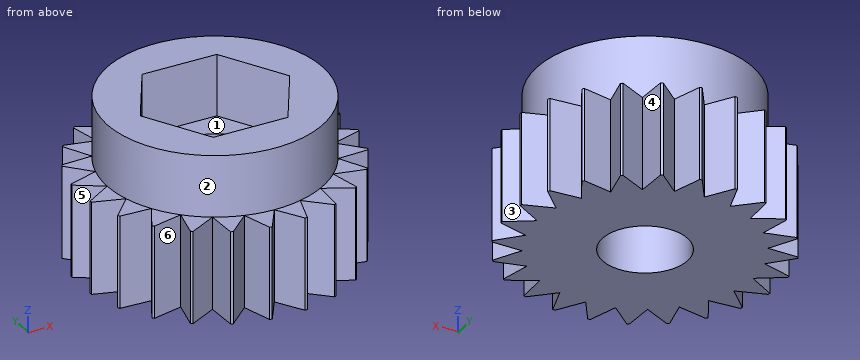
```python
from build123d import *

# Parameters (mm, degrees)
F3_DEPTH = 2.54
F4_R     = 6.6719294198
F5_DEPTH = 25.4


with BuildPart() as f1:
    # F0 (on Front) → F1 (revolve)
    with BuildSketch(Plane.XZ):
        Polygon((-5.56, -6.35), (-1.75, -6.35), (-1.75, 0), (-4.445, 0), (-4.445, -2.54), (-5.56, -2.54), align=None)
    revolve(axis=Axis((0, 0, -3.175), (0, 0, -1)))

    # F2 (on face) → F3 (cut)
    with BuildSketch(Plane.XY):
        Polygon((1.5397931679, 2.667), (-1.5397931679, 2.667), (-3.0795863359, 0), (-1.5397931679, -2.667), (1.5397931679, -2.667), (3.0795863359, 0), align=None)
    extrude(amount=-F3_DEPTH, mode=Mode.SUBTRACT)

    # F4 (on face) → F5 (cut)
    with BuildSketch(Plane.XY.offset(-2.54)):
        Circle(F4_R)
        with BuildLine():
            ThreePointArc((-0.7741932024, 5.5058355302), (-0.7257256287, 5.5124334292), (-0.6772018857, 5.5186046793))
            ThreePointArc((-0.6772018857, 5.5186046793), (0, 5.56), (0.6772018857, 5.5186046793))
            ThreePointArc((0.6772018857, 5.5186046793), (0.7257256287, 5.5124334292), (0.7741932024, 5.5058355302))
            ThreePointArc((0.7741932024, 5.5058355302), (1.4390338908, 5.3705475942), (2.0824467844, 5.1552900394))
            ThreePointArc((2.0824467844, 5.1552900394), (2.1277198839, 5.1367702008), (2.1728283032, 5.1178527885))
            ThreePointArc((2.1728283032, 5.1178527885), (2.78, 4.815101245), (3.3457763761, 4.4406509029))
            ThreePointArc((3.3457763761, 4.4406509029), (3.3847135453, 4.411044572), (3.4233887458, 4.381096837))
            ThreePointArc((3.4233887458, 4.381096837), (3.9315137034, 3.9315137034), (4.381096837, 3.4233887458))
            ThreePointArc((4.381096837, 3.4233887458), (4.411044572, 3.3847135453), (4.4406509029, 3.3457763761))
            ThreePointArc((4.4406509029, 3.3457763761), (4.815101245, 2.78), (5.1178527885, 2.1728283032))
            ThreePointArc((5.1178527885, 2.1728283032), (5.1367702008, 2.1277198839), (5.1552900394, 2.0824467844))
            ThreePointArc((5.1552900394, 2.0824467844), (5.3705475942, 1.4390338908), (5.5058355302, 0.7741932024))
            ThreePointArc((5.5058355302, 0.7741932024), (5.5124334292, 0.7257256287), (5.5186046793, 0.6772018857))
            ThreePointArc((5.5186046793, 0.6772018857), (5.5496415207, 0.339232946), (5.56, 0))
            ThreePointArc((5.56, 0), (5.5496415207, -0.339232946), (5.5186046793, -0.6772018857))
            ThreePointArc((5.5186046793, -0.6772018857), (5.5124334292, -0.7257256287), (5.5058355302, -0.7741932024))
            ThreePointArc((5.5058355302, -0.7741932024), (5.3705475942, -1.4390338908), (5.1552900394, -2.0824467844))
            ThreePointArc((5.1552900394, -2.0824467844), (5.1367702008, -2.1277198839), (5.1178527885, -2.1728283032))
            ThreePointArc((5.1178527885, -2.1728283032), (4.815101245, -2.78), (4.4406509029, -3.3457763761))
            ThreePointArc((4.4406509029, -3.3457763761), (4.411044572, -3.3847135453), (4.381096837, -3.4233887458))
            ThreePointArc((4.381096837, -3.4233887458), (3.9315137034, -3.9315137034), (3.4233887458, -4.381096837))
            ThreePointArc((3.4233887458, -4.381096837), (3.3847135453, -4.411044572), (3.3457763761, -4.4406509029))
            ThreePointArc((3.3457763761, -4.4406509029), (2.78, -4.815101245), (2.1728283032, -5.1178527885))
            ThreePointArc((2.1728283032, -5.1178527885), (2.1277198839, -5.1367702008), (2.0824467844, -5.1552900394))
            ThreePointArc((2.0824467844, -5.1552900394), (1.4390338908, -5.3705475942), (0.7741932024, -5.5058355302))
            ThreePointArc((0.7741932024, -5.5058355302), (0.7257256287, -5.5124334292), (0.6772018857, -5.5186046793))
            ThreePointArc((0.6772018857, -5.5186046793), (0, -5.56), (-0.6772018857, -5.5186046793))
            ThreePointArc((-0.6772018857, -5.5186046793), (-0.7257256287, -5.5124334292), (-0.7741932024, -5.5058355302))
            ThreePointArc((-0.7741932024, -5.5058355302), (-1.4390338908, -5.3705475942), (-2.0824467844, -5.1552900394))
            ThreePointArc((-2.0824467844, -5.1552900394), (-2.1277198839, -5.1367702008), (-2.1728283032, -5.1178527885))
            ThreePointArc((-2.1728283032, -5.1178527885), (-2.78, -4.815101245), (-3.3457763761, -4.4406509029))
            ThreePointArc((-3.3457763761, -4.4406509029), (-3.3847135453, -4.411044572), (-3.4233887458, -4.381096837))
            ThreePointArc((-3.4233887458, -4.381096837), (-3.9315137034, -3.9315137034), (-4.381096837, -3.4233887458))
            ThreePointArc((-4.381096837, -3.4233887458), (-4.411044572, -3.3847135453), (-4.4406509029, -3.3457763761))
            ThreePointArc((-4.4406509029, -3.3457763761), (-4.815101245, -2.78), (-5.1178527885, -2.1728283032))
            ThreePointArc((-5.1178527885, -2.1728283032), (-5.1367702008, -2.1277198839), (-5.1552900394, -2.0824467844))
            ThreePointArc((-5.1552900394, -2.0824467844), (-5.3705475942, -1.4390338908), (-5.5058355302, -0.7741932024))
            ThreePointArc((-5.5058355302, -0.7741932024), (-5.5124334292, -0.7257256287), (-5.5186046793, -0.6772018857))
            ThreePointArc((-5.5186046793, -0.6772018857), (-5.56, 0), (-5.5186046793, 0.6772018857))
            ThreePointArc((-5.5186046793, 0.6772018857), (-5.5124334292, 0.7257256287), (-5.5058355302, 0.7741932024))
            ThreePointArc((-5.5058355302, 0.7741932024), (-5.3705475942, 1.4390338908), (-5.1552900394, 2.0824467844))
            ThreePointArc((-5.1552900394, 2.0824467844), (-5.1367702008, 2.1277198839), (-5.1178527885, 2.1728283032))
            ThreePointArc((-5.1178527885, 2.1728283032), (-4.815101245, 2.78), (-4.4406509029, 3.3457763761))
            ThreePointArc((-4.4406509029, 3.3457763761), (-4.411044572, 3.3847135453), (-4.381096837, 3.4233887458))
            ThreePointArc((-4.381096837, 3.4233887458), (-3.9315137034, 3.9315137034), (-3.4233887458, 4.381096837))
            ThreePointArc((-3.4233887458, 4.381096837), (-3.3847135453, 4.411044572), (-3.3457763761, 4.4406509029))
            ThreePointArc((-3.3457763761, 4.4406509029), (-2.78, 4.815101245), (-2.1728283032, 5.1178527885))
            ThreePointArc((-2.1728283032, 5.1178527885), (-2.1277198839, 5.1367702008), (-2.0824467844, 5.1552900394))
            ThreePointArc((-2.0824467844, 5.1552900394), (-1.4390338908, 5.3705475942), (-0.7741932024, 5.5058355302))
        make_face(mode=Mode.SUBTRACT)
        with BuildLine():
            Line((-5.1178527885, 2.1728283032), (-3.8494829198, 2.2225))
            Line((-3.8494829198, 2.2225), (-4.4406509029, 3.3457763761))
            ThreePointArc((-4.4406509029, 3.3457763761), (-4.815101245, 2.78), (-5.1178527885, 2.1728283032))
        make_face()
        with BuildLine():
            Line((-4.381096837, 3.4233887458), (-3.1430896424, 3.1430896424))
            Line((-3.1430896424, 3.1430896424), (-3.4233887458, 4.381096837))
            ThreePointArc((-3.4233887458, 4.381096837), (-3.9315137034, 3.9315137034), (-4.381096837, 3.4233887458))
        make_face()
        with BuildLine():
            Line((-3.3457763761, 4.4406509029), (-2.2225, 3.8494829198))
            Line((-2.2225, 3.8494829198), (-2.1728283032, 5.1178527885))
            ThreePointArc((-2.1728283032, 5.1178527885), (-2.78, 4.815101245), (-3.3457763761, 4.4406509029))
        make_face()
        with BuildLine():
            Line((-2.0824467844, 5.1552900394), (-1.1504506555, 4.2935402979))
            Line((-1.1504506555, 4.2935402979), (-0.7741932024, 5.5058355302))
            ThreePointArc((-0.7741932024, 5.5058355302), (-1.4390338908, 5.3705475942), (-2.0824467844, 5.1552900394))
        make_face()
        with BuildLine():
            Line((-5.5058355302, 0.7741932024), (-4.2935402979, 1.1504506555))
            Line((-4.2935402979, 1.1504506555), (-5.1552900394, 2.0824467844))
            ThreePointArc((-5.1552900394, 2.0824467844), (-5.3705475942, 1.4390338908), (-5.5058355302, 0.7741932024))
        make_face()
        with BuildLine():
            Line((-5.5186046793, -0.6772018857), (-4.445, 0))
            Line((-4.445, 0), (-5.5186046793, 0.6772018857))
            ThreePointArc((-5.5186046793, 0.6772018857), (-5.56, 0), (-5.5186046793, -0.6772018857))
        make_face()
        with BuildLine():
            Line((-5.1552900394, -2.0824467844), (-4.2935402979, -1.1504506555))
            Line((-4.2935402979, -1.1504506555), (-5.5058355302, -0.7741932024))
            ThreePointArc((-5.5058355302, -0.7741932024), (-5.3705475942, -1.4390338908), (-5.1552900394, -2.0824467844))
        make_face()
        with BuildLine():
            Line((-4.4406509029, -3.3457763761), (-3.8494829198, -2.2225))
            Line((-3.8494829198, -2.2225), (-5.1178527885, -2.1728283032))
            ThreePointArc((-5.1178527885, -2.1728283032), (-4.815101245, -2.78), (-4.4406509029, -3.3457763761))
        make_face()
        with BuildLine():
            Line((-3.4233887458, -4.381096837), (-3.1430896424, -3.1430896424))
            Line((-3.1430896424, -3.1430896424), (-4.381096837, -3.4233887458))
            ThreePointArc((-4.381096837, -3.4233887458), (-3.9315137034, -3.9315137034), (-3.4233887458, -4.381096837))
        make_face()
        with BuildLine():
            Line((-2.1728283032, -5.1178527885), (-2.2225, -3.8494829198))
            Line((-2.2225, -3.8494829198), (-3.3457763761, -4.4406509029))
            ThreePointArc((-3.3457763761, -4.4406509029), (-2.78, -4.815101245), (-2.1728283032, -5.1178527885))
        make_face()
        with BuildLine():
            Line((-0.7741932024, -5.5058355302), (-1.1504506555, -4.2935402979))
            Line((-1.1504506555, -4.2935402979), (-2.0824467844, -5.1552900394))
            ThreePointArc((-2.0824467844, -5.1552900394), (-1.4390338908, -5.3705475942), (-0.7741932024, -5.5058355302))
        make_face()
        with BuildLine():
            Line((0.6772018857, -5.5186046793), (0, -4.445))
            Line((0, -4.445), (-0.6772018857, -5.5186046793))
            ThreePointArc((-0.6772018857, -5.5186046793), (0, -5.56), (0.6772018857, -5.5186046793))
        make_face()
        with BuildLine():
            Line((2.0824467844, -5.1552900394), (1.1504506555, -4.2935402979))
            Line((1.1504506555, -4.2935402979), (0.7741932024, -5.5058355302))
            ThreePointArc((0.7741932024, -5.5058355302), (1.4390338908, -5.3705475942), (2.0824467844, -5.1552900394))
        make_face()
        with BuildLine():
            Line((3.3457763761, -4.4406509029), (2.2225, -3.8494829198))
            Line((2.2225, -3.8494829198), (2.1728283032, -5.1178527885))
            ThreePointArc((2.1728283032, -5.1178527885), (2.78, -4.815101245), (3.3457763761, -4.4406509029))
        make_face()
        with BuildLine():
            Line((4.381096837, -3.4233887458), (3.1430896424, -3.1430896424))
            Line((3.1430896424, -3.1430896424), (3.4233887458, -4.381096837))
            ThreePointArc((3.4233887458, -4.381096837), (3.9315137034, -3.9315137034), (4.381096837, -3.4233887458))
        make_face()
        with BuildLine():
            Line((5.1178527885, -2.1728283032), (3.8494829198, -2.2225))
            Line((3.8494829198, -2.2225), (4.4406509029, -3.3457763761))
            ThreePointArc((4.4406509029, -3.3457763761), (4.815101245, -2.78), (5.1178527885, -2.1728283032))
        make_face()
        with BuildLine():
            Line((5.5058355302, -0.7741932024), (4.2935402979, -1.1504506555))
            Line((4.2935402979, -1.1504506555), (5.1552900394, -2.0824467844))
            ThreePointArc((5.1552900394, -2.0824467844), (5.3705475942, -1.4390338908), (5.5058355302, -0.7741932024))
        make_face()
        with BuildLine():
            Line((5.5186046793, 0.6772018857), (4.445, 0))
            Line((4.445, 0), (5.5186046793, -0.6772018857))
            ThreePointArc((5.5186046793, -0.6772018857), (5.5496415207, -0.339232946), (5.56, 0))
            ThreePointArc((5.56, 0), (5.5496415207, 0.339232946), (5.5186046793, 0.6772018857))
        make_face()
        with BuildLine():
            Line((5.1552900394, 2.0824467844), (4.2935402979, 1.1504506555))
            Line((4.2935402979, 1.1504506555), (5.5058355302, 0.7741932024))
            ThreePointArc((5.5058355302, 0.7741932024), (5.3705475942, 1.4390338908), (5.1552900394, 2.0824467844))
        make_face()
        with BuildLine():
            Line((4.4406509029, 3.3457763761), (3.8494829198, 2.2225))
            Line((3.8494829198, 2.2225), (5.1178527885, 2.1728283032))
            ThreePointArc((5.1178527885, 2.1728283032), (4.815101245, 2.78), (4.4406509029, 3.3457763761))
        make_face()
        with BuildLine():
            Line((3.4233887458, 4.381096837), (3.1430896424, 3.1430896424))
            Line((3.1430896424, 3.1430896424), (4.381096837, 3.4233887458))
            ThreePointArc((4.381096837, 3.4233887458), (3.9315137034, 3.9315137034), (3.4233887458, 4.381096837))
        make_face()
        with BuildLine():
            Line((2.1728283032, 5.1178527885), (2.2225, 3.8494829198))
            Line((2.2225, 3.8494829198), (3.3457763761, 4.4406509029))
            ThreePointArc((3.3457763761, 4.4406509029), (2.78, 4.815101245), (2.1728283032, 5.1178527885))
        make_face()
        with BuildLine():
            Line((0.7741932024, 5.5058355302), (1.1504506555, 4.2935402979))
            Line((1.1504506555, 4.2935402979), (2.0824467844, 5.1552900394))
            ThreePointArc((2.0824467844, 5.1552900394), (1.4390338908, 5.3705475942), (0.7741932024, 5.5058355302))
        make_face()
        with BuildLine():
            Line((-0.6772018857, 5.5186046793), (0, 4.445))
            Line((0, 4.445), (0.6772018857, 5.5186046793))
            ThreePointArc((0.6772018857, 5.5186046793), (0, 5.56), (-0.6772018857, 5.5186046793))
        make_face()
    extrude(amount=-F5_DEPTH, mode=Mode.SUBTRACT)


solid = f1.part
```
Part model, mm, in its own coordinate system. Face numbers are marked on the shaded views. A direction names the side the tool comes from. Round coordinates to 2 decimals unless told otherwise and drop trailing zeros. Loops run counter-clockwise (first coordinate to the right, second up) from the corner with the lowest first, then second, coordinate; pieces in that order, holes last. Notation, with made-up numbers: (31.5, 20) -> (88.5, 20) arc R23 cw to (88.5, 41) -> close; hole circle Ø11 at (70, 34.25). An arc over 180 degrees is marked (long way). Use a Markdown table: item, result.
1) Cut at B-B, the plane y = 1. List the corners of the cut face in (x, z).
The answers:
| item | result |
|---|---|
| outline | (-4.78, -6.35) -> (-1.44, -6.35) -> (-1.44, -2.54) -> (-2.5, -2.54) -> (-2.5, 0) -> (-4.33, 0) -> (-4.33, -2.54) -> (-4.78, -2.54) -> close; (1.44, -6.35) -> (4.78, -6.35) -> (4.78, -2.54) -> (4.33, -2.54) -> (4.33, 0) -> (2.5, 0) -> (2.5, -2.54) -> (1.44, -2.54) -> close |
2) Drop flat-ended pins along their axis: pin 1 Ø1 at (x, y) = (4, 2.5) entering from +Z; pin 2 Ø0.6 at (x, y) = (-4, -3) entering from +Z; pin 3 Ø0.8 at (x, z) = (0, -1.5) entering from -Y (3 decimals); pin 4 Ø2 at (y, z) = (-3.5, -1) entering from -X. Give the stop position or say it passes through.
The answers:
| item | result |
|---|---|
| pin 1 | stops at z = 0 |
| pin 2 | stops at z = -2.54 |
| pin 3 | stops at y = -4.445 |
| pin 4 | stops at x = -3.68 |
3) Tool access for the marked faces 4, 5 and 6: list every direction of +Z, -Z, +X, -X, +Y, -Y with a clear straight run to the whole face (end or side of a thin tool).
The answers:
| item | result |
|---|---|
| face 4 | +Z, -Z, +Y |
| face 5 | +Z, -Z, -X |
| face 6 | +Z, -Z |
4) Probe line 1 (Y direction, x = -4, z = -2.75); line 2 (Z direction, x = -0.25, y = 4.75); line 3 (Y direction, x = -5, z = -4.5). List the from-to ranges inside material, lowest first. Write a range as [from, to].
The answers:
| item | result |
|---|---|
| line 1 | y = [-3.34, -2.51], [-2.22, 2.22], [2.51, 3.34] |
| line 2 | z = [-6.35, -2.54] |
| line 3 | y = [-2.18, -1.91], [-0.93, -0.35], [0.35, 0.93], [1.91, 2.18] |
5) Cut at A-A, the plane z = -1. List the corners of the cut face in (x, y) (3 decimals).
The answers:
| item | result |
|---|---|
| outline | circle Ø8.89 at (0, 0); hole (-3.08, 0) -> (-1.54, -2.667) -> (1.54, -2.667) -> (3.08, 0) -> (1.54, 2.667) -> (-1.54, 2.667) -> close |
6) Pull direction X, two halves, no side cores. Call the marked faces 1, 2 and 3: pulls with the +X half, pulls with the -X half, needs draft (parallel to the pull), parting line crosses it, or undercut.
The answers:
| item | result |
|---|---|
| face 1 | undercut |
| face 2 | parting line crosses it |
| face 3 | pulls with the +X half |
